from build123d import *

# Parameters (mm, degrees)
SKETCH1_W                                      = 55.88
SKETCH1_H                                      = 55.88
BOSS_EXTRUDE1_DEPTH                            = 4
CBORE_FOR_4_BUTTON_HEAD_CAP_SCREW1_D           = 3.2639
CBORE_FOR_4_BUTTON_HEAD_CAP_SCREW1_CBORE_D     = 6.35
CBORE_FOR_4_BUTTON_HEAD_CAP_SCREW1_CBORE_DEPTH = 1.4986
SKETCH4_W                                      = 55.88
SKETCH4_H                                      = 8.184570626
BOSS_EXTRUDE2_DEPTH                            = 2.54
SKETCH5_W                                      = 55.88
SKETCH5_H                                      = 4.348891515
CUT_EXTRUDE1_DEPTH                             = 0.762


with BuildPart() as part:
    # Sketch1 → Boss-Extrude1 (new body)
    with BuildSketch(Plane(origin=(0, 0, 0), x_dir=(1, 0, 0), z_dir=(0, 1, 0))):
        Rectangle(SKETCH1_W, SKETCH1_H)
    extrude(amount=BOSS_EXTRUDE1_DEPTH)

    # CBORE for #4 Button Head Cap Screw1 (through all)
    with Locations(Plane(origin=(0, 4, 0), x_dir=(1, 0, 0), z_dir=(0, 1, 0))):
        with Locations((-24.13, 22.86), (24.13, 22.86), (24.13, -22.86), (-24.13, -22.86)):
            CounterBoreHole(CBORE_FOR_4_BUTTON_HEAD_CAP_SCREW1_D / 2, CBORE_FOR_4_BUTTON_HEAD_CAP_SCREW1_CBORE_D / 2, CBORE_FOR_4_BUTTON_HEAD_CAP_SCREW1_CBORE_DEPTH)

    # Sketch4 → Boss-Extrude2 (add)
    with BuildSketch(Plane.XY.offset(27.94)):
        with Locations((0, -0.092285313)):
            Rectangle(SKETCH4_W, SKETCH4_H)
    extrude(amount=BOSS_EXTRUDE2_DEPTH)

    # Sketch5 → Cut-Extrude1 (cut)
    with BuildSketch(Plane(origin=(0, 0, 27.94), x_dir=(-1, 0, 0), z_dir=(0, 0, -1))):
        with Locations((0, -2.010124869)):
            Rectangle(SKETCH5_W, SKETCH5_H)
    extrude(amount=-CUT_EXTRUDE1_DEPTH, mode=Mode.SUBTRACT)


solid = part.part
The listing builds one solid part. Answer for the finished solid, in the listing's coordinates (mm). A direction names the side the tool comes from. Coordinates: 2 decimals unless noted, no trailing zeros. Loops run counter-clockwise (first coordinate to the right, second up) from the corner with the lowest first, then second, coordinate; pieces in that order, holes last.
1) Find section D-D on x = -19.5. Write down the section's boundary in (y, z).
2) Find section C-C on y = -2. Write down the section's boundary in (x, z).
3) Find section A-A on x = 24.13. Write down the section's boundary in (y, z) (3 decimals).
4) Flat-ended cylindrical pins translate along their axes: pin 1 Ø7 at (x, z) = (24, 24) entering from +Y; pin 2 Ø7.5 at (x, z) = (24.13, 22.86) entering from -Y; pin 3 Ø3 at (x, y) = (-16.5, -2) entering from -Z; pin 4 Ø4 at (x, z) = (-24.13, 22.86) entering from +Y. Find the tip coordinate at first contact, or state that the pin passes through.
5) Find section B-B on z = -22.86. Write down the section's boundary in (x, y) (3 decimals).
6) Find the intervals of material crossed by L1, parallel to Z at x = -24.13, y = 3 (3 decimals); L2, parallel to X at y = 0.65, z = 22.86; L3, parallel to Z at x = 24.13, y = 0.5, in increasing order.
7) A tool of negligible diameter and unlimited length cuts with its end or side. For faces 4 (the face through (24.484, 1.233, 24.453)), 5 (the face through (25, 2.501, -21)), from which of +Z, -Z, +X, -X, +Y, -Y can it reach the whole face along a straight path? Write none if from no direction.
8) Determine the mould class of faces 1 (the face through (0, 2, -27.94)), 2 (the face through (-27.94, 3, 1)), 3 (the face through (-25, 2.501, 21)) for opening direction Z: pulls with the +Z half, pulls with the -Z half, needs draft (parallel to the pull), parting line crosses it, or undercut.
Values:
1. outline: (-4.18, 28.7) - (0.16, 28.7) - (0.16, 27.94) - (0, 27.94) - (0, -27.94) - (4, -27.94) - (4, 30.48) - (-4.18, 30.48) - close
2. outline: (-27.94, 28.7) - (27.94, 28.7) - (27.94, 30.48) - (-27.94, 30.48) - close
3. outline: (-4.185, 28.702) - (0.164, 28.702) - (0.164, 27.94) - (0, 27.94) - (0, 24.492) - (2.501, 24.492) - (2.501, 26.035) - (4, 26.035) - (4, 30.48) - (-4.185, 30.48) - close; (0, -27.94) - (4, -27.94) - (4, -26.035) - (2.501, -26.035) - (2.501, -24.492) - (0, -24.492) - close; (0, -21.228) - (2.501, -21.228) - (2.501, -19.685) - (4, -19.685) - (4, 19.685) - (2.501, 19.685) - (2.501, 21.228) - (0, 21.228) - close
4. pin 1: stops at y = 4
4. pin 2: stops at y = 0
4. pin 3: stops at z = 28.7
4. pin 4: stops at y = 2.5
5. outline: (-27.94, 0) - (-25.762, 0) - (-25.762, 2.501) - (-27.305, 2.501) - (-27.305, 4) - (-27.94, 4) - close; (-22.498, 0) - (22.498, 0) - (22.498, 2.501) - (20.955, 2.501) - (20.955, 4) - (-20.955, 4) - (-20.955, 2.501) - (-22.498, 2.501) - close; (25.762, 0) - (27.94, 0) - (27.94, 4) - (27.305, 4) - (27.305, 2.501) - (25.762, 2.501) - close
6. L1: z = -27.94 to -26.035, -19.685 to 19.685, 26.035 to 30.48
6. L2: x = -27.94 to -25.76, -22.5 to 22.5, 25.76 to 27.94
6. L3: z = -27.94 to -24.49, -21.23 to 21.23, 24.49 to 30.48
7. face 4: +Y, -Y
7. face 5: +Y
8. face 1: pulls with the -Z half
8. face 2: needs draft
8. face 3: undercut
